from build123d import *

# Parameters (mm, degrees)
SKETCH1_W                       = 9
SKETCH1_H                       = 26.38
SKETCH1_R                       = 1.9
BODY_MOUNT_DEPTH                = 3
SKETCH2_W                       = 5
SKETCH2_H                       = 3
BOSS_EXTRUDE2_DEPTH             = 25
SKETCH3_W                       = 5
SKETCH3_H                       = 5
BOSS_EXTRUDE3_DEPTH             = 20
SKETCH4_R                       = 1.5
CUT_EXTRUDE1_DEPTH              = 20
BOSS_EXTRUDE4_REACH             = 39.616
BOSS_EXTRUDE4_DIRECTION_2_REACH = 39.616
FILLET2_R                       = 5


with BuildPart() as part:
    # Sketch1 → body mount (new body)
    with BuildSketch(Plane(origin=(0, 0, 0), x_dir=(1, 0, 0), z_dir=(0, 1, 0))):
        with Locations((-0.5, 8.155)):
            Rectangle(SKETCH1_W, SKETCH1_H)
        with Locations(Location((0, 0, 0), (0, 0, 270))):
            Circle(SKETCH1_R, mode=Mode.SUBTRACT)
        with Locations(Location((0, 16.31, 0), (0, 0, 270))):
            Circle(SKETCH1_R, mode=Mode.SUBTRACT)
    extrude(amount=BODY_MOUNT_DEPTH)

    # Sketch2 → Boss-Extrude2 (add)
    with BuildSketch(Plane(origin=(4, 0, 0), x_dir=(0, 0, -1), z_dir=(1, 0, 0))):
        with Locations((8.155, 1.5)):
            Rectangle(SKETCH2_W, SKETCH2_H)
    extrude(amount=BOSS_EXTRUDE2_DEPTH)

    # Sketch3 → Boss-Extrude3 (add)
    with BuildSketch(Plane.XZ):
        with Locations((26.5, -8.155)):
            Rectangle(SKETCH3_W, SKETCH3_H)
    extrude(amount=BOSS_EXTRUDE3_DEPTH)

    # Sketch4 → Cut-Extrude1 (cut)
    with BuildSketch(Plane(origin=(0, 0, -10.655), x_dir=(-1, 0, 0), z_dir=(0, 0, -1))):
        with Locations((-26.5, -17)):
            Circle(SKETCH4_R)
        with Locations((-26.5, -7.5)):
            Circle(SKETCH4_R)
    extrude(amount=-CUT_EXTRUDE1_DEPTH, mode=Mode.SUBTRACT)

    # Boss-Extrude4: up to this face of the body (flat: up to its plane)
    boss_extrude4_end = Plane(part.part.faces().sort_by_distance((16.5, 2.660294245, -10.655))[0])
    # Sketch5 → Boss-Extrude4 (add, up to the picked face)
    with BuildSketch(Plane(origin=(0, 0, -8.155), x_dir=(-1, 0, 0), z_dir=(0, 0, -1)), mode=Mode.PRIVATE) as boss_extrude4_sk1:
        Polygon((-24, -10.415369352), (-9.210305315, 0), (-4, 0), (-24, -14.084630648), align=None)
    boss_extrude4_tool1 = split(extrude(boss_extrude4_sk1.sketch, amount=BOSS_EXTRUDE4_REACH, mode=Mode.PRIVATE), bisect_by=boss_extrude4_end, keep=Keep.BOTH, mode=Mode.PRIVATE)
    add(boss_extrude4_tool1.solids().sort_by(Axis((15.237549, -6.170794, -8.155), (0, 0, -1)))[0])

    # Boss-Extrude4 direction 2: up to this face of the body (flat: up to its plane)
    boss_extrude4_direction_2_end = Plane(part.part.faces().sort_by_distance((14, 0.339705755, -5.655))[0])
    # Sketch5 → Boss-Extrude4 direction 2 (add, up to the picked face)
    with BuildSketch(Plane(origin=(0, 0, -8.155), x_dir=(-1, 0, 0), z_dir=(0, 0, -1)), mode=Mode.PRIVATE) as boss_extrude4_direction_2_sk1:
        Polygon((-24, -10.415369352), (-9.210305315, 0), (-4, 0), (-24, -14.084630648), align=None)
    boss_extrude4_direction_2_tool1 = split(extrude(boss_extrude4_direction_2_sk1.sketch, amount=-BOSS_EXTRUDE4_DIRECTION_2_REACH, mode=Mode.PRIVATE), bisect_by=boss_extrude4_direction_2_end, keep=Keep.BOTH, mode=Mode.PRIVATE)
    add(boss_extrude4_direction_2_tool1.solids().sort_by(Axis((15.237549, -6.170794, -8.155), (0, 0, 1)))[0])

    # Fillet2
    # the kernel refuses this fillet: 5 mm, written as the material it adds along each edge
    with BuildSketch(Plane(origin=(4, 3, -10.655), x_dir=(0, 0, -1), z_dir=(0, -1, 0))) as fillet2_piece_1_section:
        with BuildLine():
            CenterArc((FILLET2_R, FILLET2_R), FILLET2_R, 180, 90)
            Line((0, FILLET2_R), (0, 0))
            Line((0, 0), (FILLET2_R, 0))
        make_face()
    fillet2_piece_1 = extrude(amount=3, mode=Mode.PRIVATE)
    fillet2_piece_1 = split(fillet2_piece_1, bisect_by=Plane(origin=(4.050655402, -0.035673131, -11.785736825), z_dir=(0.5757819971310116, 0.8176032606220598, 0)), keep=Keep.TOP, mode=Mode.PRIVATE)
    add(fillet2_piece_1)
    with BuildSketch(Plane(origin=(4, 3, -10.655), x_dir=(0, 0, -1), z_dir=(0, -1, 0))) as fillet2_piece_2_section:
        with BuildLine():
            CenterArc((FILLET2_R, FILLET2_R), FILLET2_R, 180, 90)
            Line((0, FILLET2_R), (0, 0))
            Line((0, 0), (FILLET2_R, 0))
        make_face()
    fillet2_piece_2 = extrude(amount=15.5, mode=Mode.PRIVATE)
    fillet2_piece_2 = split(fillet2_piece_2, bisect_by=Plane(origin=(6.150590259, 0, -11.187362576), z_dir=(0, -1, 0)), keep=Keep.TOP, mode=Mode.PRIVATE)
    fillet2_piece_2 = split(fillet2_piece_2, bisect_by=Plane(origin=(5.79410314, -1.263464003, -11.187362576), z_dir=(0.5757819971310116, 0.8176032606220598, 0)), keep=Keep.TOP, mode=Mode.PRIVATE)
    add(fillet2_piece_2)
    with BuildSketch(Plane(origin=(4, -12.5, -5.655), x_dir=(1, 0, 0), z_dir=(0, 1, 0))) as fillet2_piece_3_section:
        with BuildLine():
            CenterArc((FILLET2_R, -FILLET2_R), FILLET2_R, 90, 90)
            Line((0, -FILLET2_R), (0, 0))
            Line((0, 0), (FILLET2_R, 0))
        make_face()
    fillet2_piece_3 = extrude(amount=15.5, mode=Mode.PRIVATE)
    fillet2_piece_3 = split(fillet2_piece_3, bisect_by=Plane(origin=(5.79410314, -1.263464003, -5.122637424), z_dir=(0.5757819971310116, 0.8176032606220598, 0)), keep=Keep.TOP, mode=Mode.PRIVATE)
    fillet2_piece_3 = split(fillet2_piece_3, bisect_by=Plane(origin=(6.150590259, 0, -5.122637424), z_dir=(0, -1, 0)), keep=Keep.TOP, mode=Mode.PRIVATE)
    add(fillet2_piece_3)
    with BuildSketch(Plane(origin=(4, 0, -5.655), x_dir=(1, 0, 0), z_dir=(0, 1, 0))) as fillet2_piece_4_section:
        with BuildLine():
            CenterArc((FILLET2_R, -FILLET2_R), FILLET2_R, 90, 90)
            Line((0, -FILLET2_R), (0, 0))
            Line((0, 0), (FILLET2_R, 0))
        make_face()
    fillet2_piece_4 = extrude(amount=3, mode=Mode.PRIVATE)
    fillet2_piece_4 = split(fillet2_piece_4, bisect_by=Plane(origin=(4.050655402, -0.035673131, -4.524263175), z_dir=(0.5757819971310116, 0.8176032606220598, 0)), keep=Keep.TOP, mode=Mode.PRIVATE)
    add(fillet2_piece_4)


solid = part.part
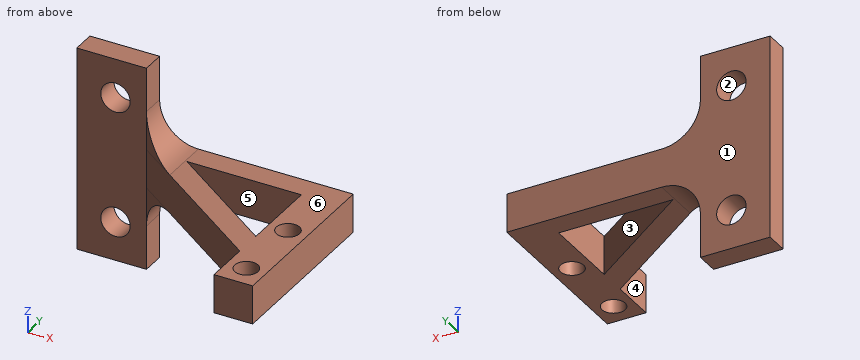
Check sheet for the modelled part. Datum: model origin and axes. Units: mm. Face numbers are marked on the shaded views. A direction names the side the tool comes from. Round coordinates to 2 decimals unless told otherwise and drop trailing zeros. Order: outer loops, then holes, each group sorted by start corner. A loop starts at its lowest first (then second) coordinate and runs counter-clockwise, first axis right, second up.
(1) Draft check along Y on the marked faces 1, 2 and 3. Enter one of: pulls with the +Y half, pulls with the -Y half, needs draft (parallel to the pull), parting line crosses it, or undercut.
(2) Cross-section at C-C, the plane y = -17. Enter the section's corners in (x, z) (3 decimals), and give its area (3 significant figures).
(3) Go/stop test with flat-tipped pins: P1, Ø10, axis at x = -1.5, z = -17, coming from the -Y side; P2, Ø8, axis at x = 8, z = -9.5, coming from the -Y side; P3, Ø2.5, axis at y = -18.5, z = -7, coming from the -X side. Record where each tip stops, or that it passes through.
(4) Cross-section at D-D, the plane z = 0. Enter the section's corners in (x, y).
(5) Scan lines: probe 1 along Y at (x, z) = (26.5, -9.25); probe 2 along X at (y, z) = (1.7, 0); probe 3 along X at (y, z) = (-15, -9.75). Record each from-to range of solid material in increasing order.
(6) Access from +Z, -Z, +X, -X, +Y, -Y to the whole of each face (thin tool, end or side, straight path). Record for the marked faces 4, 5 and 6.
(7) Cross-section at B-B, the plane z = -7. Enter the section's corners in (x, y).
(8) Cross-section at A-A, the plane x = 0. Enter the section's corners in (y, z) (3 decimals), and give its area (3 significant figures).
Check sheet entries:
1. face 1: pulls with the +Y half
1. face 2: needs draft
1. face 3: undercut
2. outline: (24, -10.655) - (25, -10.655) - (25, -5.655) - (24, -5.655) - close; (28, -10.655) - (29, -10.655) - (29, -5.655) - (28, -5.655) - close
2. area: 10.0 mm2
3. P1: stops at y = 0
3. P2: stops at y = -5.63
3. P3: stops at x = 24
4. outline: (-5, 0) - (-1.9, 0) - (-1.9, 3) - (-5, 3) - close; (1.9, 0) - (4, 0) - (4, 3) - (1.9, 3) - close
5. probe 1: y = -20 to -18.5, -15.5 to -9, -6 to 3
5. probe 2: x = -5 to -1.9, 1.9 to 4
5. probe 3: x = 24 to 29
6. face 4: +Z, -Z, -X, -Y
6. face 5: +Z, -Z
6. face 6: +Z, +X, +Y, -Y
7. outline: (-5, 0) - (4, 0) - (24, -14.08) - (24, -20) - (29, -20) - (29, 3) - (-5, 3) - close; hole (9.21, 0) - (24, -10.42) - (24, 0) - close; hole circle Ø3 at (26.5, -17); hole circle Ø3 at (26.5, -7.5)
8. outline: (0, -21.345) - (3, -21.345) - (3, -18.21) - (0, -18.21) - close; (0, -14.41) - (3, -14.41) - (3, -1.9) - (0, -1.9) - close; (0, 1.9) - (3, 1.9) - (3, 5.035) - (0, 5.035) - close
8. area: 56.3 mm2
